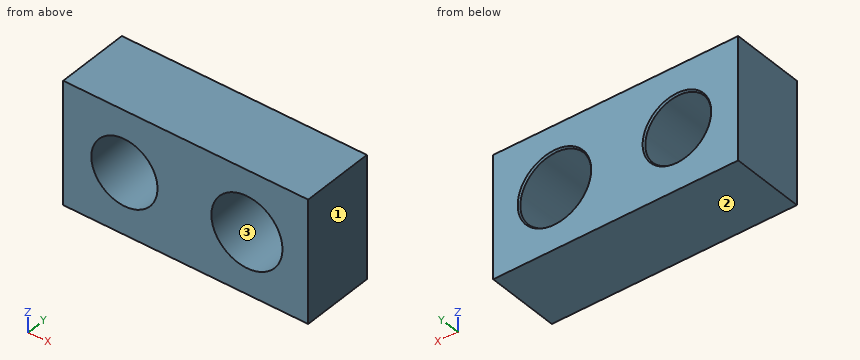
```python
from build123d import *

# Parameters (mm, degrees)
SKETCH1_W                            = 20
SKETCH1_H                            = 10
BOSS_EXTRUDE1_DEPTH                  = 6
F_5_4_5_4_DIAMETER_HOLE1_D           = 5.4
F_5_4_5_4_DIAMETER_HOLE1_CSINK_D     = 5.6
F_5_4_5_4_DIAMETER_HOLE1_CSINK_ANGLE = 70
F_5_8_5_8_DIAMETER_HOLE1_D           = 5.8
F_5_8_5_8_DIAMETER_HOLE1_CSINK_D     = 6
F_5_8_5_8_DIAMETER_HOLE1_CSINK_ANGLE = 70


with BuildPart() as part:
    # Sketch1 → Boss-Extrude1 (new body)
    with BuildSketch(Plane(origin=(0, 0, 0), x_dir=(1, 0, 0), z_dir=(0, 1, 0))):
        with Locations((10, 5)):
            Rectangle(SKETCH1_W, SKETCH1_H)
    extrude(amount=BOSS_EXTRUDE1_DEPTH)

    # Ø5.4 (5.4) Diameter Hole1 (through all)
    with Locations(Plane(origin=(0, 6, 0), x_dir=(1, 0, 0), z_dir=(0, 1, 0))):
        with Locations((5, 5)):
            CounterSinkHole(F_5_4_5_4_DIAMETER_HOLE1_D / 2, F_5_4_5_4_DIAMETER_HOLE1_CSINK_D / 2, counter_sink_angle=F_5_4_5_4_DIAMETER_HOLE1_CSINK_ANGLE)

    # Ø5.8 (5.8) Diameter Hole1 (through all)
    with Locations(Plane(origin=(0, 6, 0), x_dir=(1, 0, 0), z_dir=(0, 1, 0))):
        with Locations((15, 5)):
            CounterSinkHole(F_5_8_5_8_DIAMETER_HOLE1_D / 2, F_5_8_5_8_DIAMETER_HOLE1_CSINK_D / 2, counter_sink_angle=F_5_8_5_8_DIAMETER_HOLE1_CSINK_ANGLE)


solid = part.part
```
Here's how the part is built. I have some questions about the finished solid (model axes, mm). Face numbers are marked on the shaded views. Coordinates: 2 decimals unless noted, no trailing zeros. Write each loop counter-clockwise with the first axis right and the second up, starting at its lowest first coordinate (ties: lowest second). Pieces come first, ordered by that corner, then holes. Notation, with made-up numbers: (17.25, -5) - (23.25, -5) arc R6 cw to (23.25, 4) - close; hole circle Ø10 at (68, 43). An arc over 180 degrees is marked (long way). One line per item, written item: value.
1) I need wall thicknesses on line 1 along X through (y, z) = (4.85, -3.5) (3 decimals); line 2 along X through (y, z) = (1.5, -6); line 3 along Z through (x, y) = (15, 2). Which ranges of each line are inside material? Lowest first, please.
Model answer:
line 1: x = 0 to 2.755, 7.245 to 12.518, 17.482 to 20
line 2: x = 0 to 2.49, 7.51 to 12.28, 17.72 to 20
line 3: z = -10 to -7.9, -2.1 to 0
2) We'd pull the mould along Z, two halves only. Please class the marked faces 1, 2 and 3: pulls with the +Z half, pulls with the -Z half, needs draft (parallel to the pull), parting line crosses it, or undercut.
Model answer:
face 1: needs draft
face 2: pulls with the -Z half
face 3: undercut
3) Suppose I cut it at D-D on x = 15. Write out the boundary of the cut face in (y, z), and give its area (3 significant figures).
Model answer:
outline: (0, -10) - (6, -10) - (6, -8) - (5.86, -7.9) - (0, -7.9) - close; (0, -2.1) - (5.86, -2.1) - (6, -2) - (6, 0) - (0, 0) - close
area: 25.2 mm²
4) Suppose I cut it at A-A on x = 5. Write out the boundary of the cut face in (y, z), and give its area (3 significant figures).
Model answer:
outline: (0, -10) - (6, -10) - (6, -7.8) - (5.86, -7.7) - (0, -7.7) - close; (0, -2.3) - (5.86, -2.3) - (6, -2.2) - (6, 0) - (0, 0) - close
area: 27.6 mm²
5) Suppose I cut it at C-C on y = 3.5. Write out the boundary of the cut face in (x, z), and give its area (3 significant figures).
Model answer:
outline: (0, -10) - (20, -10) - (20, 0) - (0, 0) - close; hole circle Ø5.4 at (5, -5); hole circle Ø5.8 at (15, -5)
area: 151 mm²
6) Suppose I cut it at B-B on z = -5. Write out the boundary of the cut face in (x, y), and give its area (3 significant figures).
Model answer:
outline: (0, 0) - (2.3, 0) - (2.3, 5.86) - (2.2, 6) - (0, 6) - close; (7.7, 0) - (12.1, 0) - (12.1, 5.86) - (12, 6) - (7.8, 6) - (7.7, 5.86) - close; (17.9, 0) - (20, 0) - (20, 6) - (18, 6) - (17.9, 5.86) - close
area: 52.8 mm²
